from build123d import *

# Parameters (mm, degrees)
SKETCH2_W           = 21
SKETCH2_H           = 21
BOSS_EXTRUDE1_DEPTH = 20
SKETCH3_W           = 15
SKETCH3_H           = 15
CUT_EXTRUDE1_DEPTH  = 20
SKETCH4_W           = 4
SKETCH4_H           = 7.5
BOSS_EXTRUDE2_DEPTH = 20
FILLET2_R           = 2
SKETCH5_W           = 7
SKETCH5_H           = 32
BOSS_EXTRUDE3_DEPTH = 4
SKETCH6_W           = 3
SKETCH6_H           = 32
BOSS_EXTRUDE4_DEPTH = 70
SKETCH8_R           = 1.375
CUT_EXTRUDE2_DEPTH  = 4


with BuildPart() as part:
    # Sketch2 → Boss-Extrude1 (new body)
    with BuildSketch(Plane.XY):
        Rectangle(SKETCH2_W, SKETCH2_H)
    extrude(amount=BOSS_EXTRUDE1_DEPTH)

    # Sketch3 → Cut-Extrude1 (cut)
    with BuildSketch(Plane.XY.offset(20)):
        Rectangle(SKETCH3_W, SKETCH3_H)
    extrude(amount=-CUT_EXTRUDE1_DEPTH, mode=Mode.SUBTRACT)

    # Sketch4 → Boss-Extrude2 (add)
    with BuildSketch(Plane.ZY.offset(10.5)):
        with Locations((2, 0)):
            Rectangle(SKETCH4_W, SKETCH4_H)
    extrude(amount=BOSS_EXTRUDE2_DEPTH)

    # Fillet2
    fillet2_edges = [part.edges().sort_by_distance(p)[0] for p in [
        (-20.5, -3.75, 4),
        (-20.5, 3.75, 4),
    ]]
    fillet(fillet2_edges, radius=FILLET2_R)

    # Sketch5 → Boss-Extrude3 (add)
    with BuildSketch(Plane.ZY.offset(30.5)):
        with Locations((3.5, 0)):
            Rectangle(SKETCH5_W, SKETCH5_H)
    extrude(amount=BOSS_EXTRUDE3_DEPTH)

    # Sketch6 → Boss-Extrude4 (add)
    with BuildSketch(Plane.ZY.offset(34.5)):
        with Locations((1.5, 0)):
            Rectangle(SKETCH6_W, SKETCH6_H)
    extrude(amount=BOSS_EXTRUDE4_DEPTH)

    # Sketch8 → Cut-Extrude2 (cut)
    with BuildSketch(Plane.XY.offset(3)):
        with Locations((-39, -11.5)):
            Circle(SKETCH8_R)
        with Locations((-39, 11.5)):
            Circle(SKETCH8_R)
        with Locations((-97, -11.5)):
            Circle(SKETCH8_R)
        with Locations((-97, 11.5)):
            Circle(SKETCH8_R)
    extrude(amount=-CUT_EXTRUDE2_DEPTH, mode=Mode.SUBTRACT)


solid = part.part
Geometry check sheet. Reference: the model listing, model coordinates, mm. A direction names the side the tool comes from. Round coordinates to 2 decimals unless told otherwise and drop trailing zeros. Loops run counter-clockwise (first coordinate to the right, second up) from the corner with the lowest first, then second, coordinate; pieces in that order, holes last. Notation, with made-up numbers: (11.25, 24) - (28.25, 24) arc R17 cw to (28.25, 37) - close; hole circle Ø7 at (64.25, -39). An arc over 180 degrees is marked (long way). Answer as CSV lines item,"result".
(1) Depth check by flat-ended pin: pin 1 Ø5 at (x, z) = (-13.5, 9) entering from +Y; pin 2 Ø7.5 at (x, z) = (0.5, 10) entering from -Y; pin 3 Ø3 at (x, y) = (-20, 0.5) entering from +Z; pin 4 Ø2 at (x, z) = (-18, 0.5) entering from -Y. Enter the tip coordinate at first touch or a pass-through.
Output values:
pin 1,"passes through"
pin 2,"stops at y = -10.5"
pin 3,"stops at z = 4"
pin 4,"stops at y = -3.75"
(2) Cross-section at B-B, the plane y = 11.5. Enter the section's corners in (x, z) (3 decimals).
Output values:
outline,"(-104.5, 0) - (-98.375, 0) - (-98.375, 3) - (-104.5, 3) - close; (-95.625, 0) - (-40.375, 0) - (-40.375, 3) - (-95.625, 3) - close; (-37.625, 0) - (-30.5, 0) - (-30.5, 7) - (-34.5, 7) - (-34.5, 3) - (-37.625, 3) - close"
(3) Set-up check for faces 4 (the face through (7.5, 0, 10)), 5 (the face through (-20.64, -3.18, 3.4)), 6 (the face through (-30.5, 0.2, 4.2)), 7 (the face through (-20.64, 3.15, 3.43)): record each of +Z, -Z, +X, -X, +Y, -Y from which the full face is reachable in a straight line by a thin tool's end or side.
Output values:
face 4,"+Z, -Z"
face 5,"+Z, -Y"
face 6,"+Z"
face 7,"+Z, +Y"
(4) Release check for a two-part mould opening along X. For faces 1 (the face through (-20, 3.75, 1)), 2 (the face through (-104.5, 0, 1)), 3 (the face through (0, -10.5, 10)) record: released by +X, released by -X, zero draft, split by the parting line, or undercut.
Output values:
face 1,"undercut"
face 2,"released by -X"
face 3,"zero draft"
(5) Cross-section at D-D, the plane z = 9.25. Enter the section's corners in (x, y), and give its area (3 significant figures).
Output values:
outline,"(-10.5, -10.5) - (10.5, -10.5) - (10.5, 10.5) - (-10.5, 10.5) - close; hole (-7.5, -7.5) - (7.5, -7.5) - (7.5, 7.5) - (-7.5, 7.5) - close"
area,"216 mm²"
(6) Material ranges on line 1 along Y through (x, z) = (-97, 1.2) (3 decimals); line 2 along X through (y, z) = (-5.5, 7.75); line 3 along X through (y, z) = (-8.5, 2.5), recorded low to high.
Output values:
line 1,"y = -16 to -12.875, -10.125 to 10.125, 12.875 to 16"
line 2,"x = -10.5 to -7.5, 7.5 to 10.5"
line 3,"x = -104.5 to -30.5, -10.5 to 10.5"
(7) Cross-section at A-A, the plane x = -97. Enter the section's corners in (y, z) (3 decimals), and give its area (3 significant figures).
Output values:
outline,"(-16, 0) - (-12.875, 0) - (-12.875, 3) - (-16, 3) - close; (-10.125, 0) - (10.125, 0) - (10.125, 3) - (-10.125, 3) - close; (12.875, 0) - (16, 0) - (16, 3) - (12.875, 3) - close"
area,"79.5 mm²"
(8) Cross-section at C-C, the plane x = 0. Enter the section's corners in (y, z).
Output values:
outline,"(-10.5, 0) - (-7.5, 0) - (-7.5, 20) - (-10.5, 20) - close; (7.5, 0) - (10.5, 0) - (10.5, 20) - (7.5, 20) - close"
